Could you check a few things on this model? Use its own coordinates, in mm. A direction names the side the tool comes from. Give positions to 0.01 mm unless a question says otherwise; leave off trailing zeros. Order: outer loops, then holes, each group sorted by start corner. A loop starts at its lowest first (then second) coordinate and runs counter-clockwise, first axis right, second up. Notation, with made-up numbers: (46.25, -35) -> (92.25, -35) arc R16 ccw to (92.25, -28) -> close; hole circle Ø7 at (3.25, 25). An arc over 180 degrees is marked (long way). Answer as CSV lines item,"result". Start each with the question number.
(1) I want a section at A-A (y = 4.5). Please give me the cut outline in (x, z).
(2) Will these pins go through, and if not, where does the flat tip stop? pin 1 Ø1 at (x, y) = (-8.5, 5) entering from +Z; pin 2 Ø2 at (x, z) = (-15.25, -15.25) entering from -Y; pin 3 Ø0.7 at (x, y) = (10, -0.5) entering from -Z; pin 4 Ø6 at (x, z) = (-1.5, 5.5) entering from +Y.
(3) I want a section at C-C (y = 0). Give the number of separate pieces and of enclosed holes in the cut face, plus the area to 3 significant figures.
(4) I need wall thicknesses on L1, parallel to X at y = 2.5, z = -10; L2, parallel to X at y = -1.4, z = -10; L3, parallel to X at y = -0.2, z = -15.25. Which ranges of each line are inside material? Lowest first, please.
(5) I want a section at B-B (z = 5). Please give me the cut outline in (x, y).
(6) We'd pull the mould along Z, two halves only. Please class faces 1 (the face through (10.203, 0.024, -21.141)), 2 (the face through (9, 0, -24.5)), 3 (the face through (-12.46, 0.02, -11.44)): released by +Z, released by -Z, zero draft, split by the parting line, or undercut.
(7) On a 3-axis mill with a long thin cutter (end or side, diameter ignored), from which of +Z, -Z, +X, -X, +Y, -Y can I reach the whole of each face in a straight line? I mean faces 4 (the face through (-12, 6.7, 10)), 5 (the face through (-14, 0, -20)), 6 (the face through (10, 0, 12.85)), 7 (the face through (8.388, 4.235, 7.897)). Say none if no direction works.
```python
from build123d import *

# Parameters (mm, degrees)
BOSS_EXTRUDE1_DEPTH = 1.7
SKETCH2_R           = 1.65
CUT_EXTRUDE1_DEPTH  = 3.4
BOSS_EXTRUDE2_START = 5
SKETCH3_R           = 2.65
SKETCH3_R_2         = 1.65
BOSS_EXTRUDE2_DEPTH = 5
CUT_EXTRUDE2_START  = -0.5
CUT_EXTRUDE2_DEPTH  = 2.4


with BuildPart() as part:
    # Sketch1 → Boss-Extrude1 (new, symmetric)
    with BuildSketch(Plane(origin=(0, 0, 0), x_dir=(1, 0, 0), z_dir=(0, 1, 0))):
        with BuildLine():
            Line((-13, 20), (-15.757359313, 20))
            Line((-15.757359313, 20), (-20, 15.757359313))
            Line((-20, 15.757359313), (-20, -15.757359313))
            Line((-20, -15.757359313), (-15.757359313, -20))
            Line((-15.757359313, -20), (15.757359313, -20))
            Line((15.757359313, -20), (20, -15.757359313))
            Line((20, -15.757359313), (20, 15.757359313))
            Line((20, 15.757359313), (15.757359313, 20))
            Line((15.757359313, 20), (13, 20))
            ThreePointArc((13, 20), (10.171572875, 21.171572875), (9, 24))
            Line((9, 24), (9, 25))
            ThreePointArc((9, 25), (7.828427125, 27.828427125), (5, 29))
            Line((5, 29), (-5, 29))
            ThreePointArc((-5, 29), (-7.828427125, 27.828427125), (-9, 25))
            Line((-9, 25), (-9, 24))
            ThreePointArc((-9, 24), (-10.171572875, 21.171572875), (-13, 20))
        make_face()
    extrude(amount=BOSS_EXTRUDE1_DEPTH, both=True)

    # Sketch2 → Cut-Extrude1 (cut)
    with BuildSketch(Plane(origin=(0, 1.7, 0), x_dir=(1, 0, 0), z_dir=(0, 1, 0))):
        with Locations(Location((-10, 10, 0), (0, 0, 270))):
            Circle(SKETCH2_R)
        with Locations(Location((10, 10, 0), (0, 0, 270))):
            Circle(SKETCH2_R)
        with Locations(Location((-10, -10, 0), (0, 0, 270))):
            Circle(SKETCH2_R)
        with Locations(Location((10, -10, 0), (0, 0, 270))):
            Circle(SKETCH2_R)
        with Locations(Location((-15.25, -15.25, 0), (0, 0, 270))):
            Circle(SKETCH2_R)
        with Locations(Location((-15.25, 15.25, 0), (0, 0, 270))):
            Circle(SKETCH2_R)
        with Locations(Location((15.25, 15.25, 0), (0, 0, 270))):
            Circle(SKETCH2_R)
        with Locations(Location((15.25, -15.25, 0), (0, 0, 270))):
            Circle(SKETCH2_R)
    extrude(amount=-CUT_EXTRUDE1_DEPTH, mode=Mode.SUBTRACT)

    # Sketch3 → Boss-Extrude2 (add)
    # profile 1 of 4: a face of its own
    with BuildSketch(Plane(origin=(0, 1.7, 0), x_dir=(1, 0, 0), z_dir=(0, 1, 0)).offset(BOSS_EXTRUDE2_START)):
        with Locations(Location((-10, 10, 0), (0, 0, 270))):
            Circle(SKETCH3_R)
        with Locations(Location((-10, 10, 0), (0, 0, 270))):
            Circle(SKETCH3_R_2, mode=Mode.SUBTRACT)
    # profile 2 of 4: a face of its own
    with BuildSketch(Plane(origin=(0, 1.7, 0), x_dir=(1, 0, 0), z_dir=(0, 1, 0)).offset(BOSS_EXTRUDE2_START)):
        with Locations(Location((10, 10, 0), (0, 0, 270))):
            Circle(SKETCH3_R)
        with Locations(Location((10, 10, 0), (0, 0, 270))):
            Circle(SKETCH3_R_2, mode=Mode.SUBTRACT)
    # profile 3 of 4: a face of its own
    with BuildSketch(Plane(origin=(0, 1.7, 0), x_dir=(1, 0, 0), z_dir=(0, 1, 0)).offset(BOSS_EXTRUDE2_START)):
        with Locations(Location((10, -10, 0), (0, 0, 270))):
            Circle(SKETCH3_R)
        with Locations(Location((10, -10, 0), (0, 0, 270))):
            Circle(SKETCH3_R_2, mode=Mode.SUBTRACT)
    # profile 4 of 4: a face of its own
    with BuildSketch(Plane(origin=(0, 1.7, 0), x_dir=(1, 0, 0), z_dir=(0, 1, 0)).offset(BOSS_EXTRUDE2_START)):
        with Locations(Location((-10, -10, 0), (0, 0, 270))):
            Circle(SKETCH3_R)
        with Locations(Location((-10, -10, 0), (0, 0, 270))):
            Circle(SKETCH3_R_2, mode=Mode.SUBTRACT)
    extrude(amount=-BOSS_EXTRUDE2_DEPTH)

    # Sketch4 → Cut-Extrude2 (cut)
    with BuildSketch(Plane(origin=(0, 1.7, 0), x_dir=(1, 0, 0), z_dir=(0, 1, 0)).offset(CUT_EXTRUDE2_START)):
        Polygon((-6.709103466, 10), (-8.354551733, 12.85), (-11.645448267, 12.85), (-13.290896534, 10), (-11.645448267, 7.15), (-8.354551733, 7.15), align=None)
        Polygon((13.290896534, 10), (11.645448267, 12.85), (8.354551733, 12.85), (6.709103466, 10), (8.354551733, 7.15), (11.645448267, 7.15), align=None)
        Polygon((13.290896534, -10), (11.645448267, -7.15), (8.354551733, -7.15), (6.709103466, -10), (8.354551733, -12.85), (11.645448267, -12.85), align=None)
        Polygon((-6.709103466, -10), (-8.354551733, -7.15), (-11.645448267, -7.15), (-13.290896534, -10), (-11.645448267, -12.85), (-8.354551733, -12.85), align=None)
    extrude(amount=-CUT_EXTRUDE2_DEPTH, mode=Mode.SUBTRACT)


solid = part.part
```
Final values:
1,outline,"circle Ø5.3 at (-10, -10); circle Ø5.3 at (-10, 10); circle Ø5.3 at (10, -10); circle Ø5.3 at (10, 10); hole circle Ø3.3 at (-10, -10); hole circle Ø3.3 at (-10, 10); hole circle Ø3.3 at (10, -10); hole circle Ø3.3 at (10, 10)"
2,pin 1,"z = 12.45"
2,pin 2,"through"
2,pin 3,"z = -21.81"
2,pin 4,"y = 1.7"
3,separate pieces,"1"
3,enclosed holes,"8"
3,area,"1,580 mm²"
4,L1,"-12.65 to -11.65, -8.35 to -7.35, 7.35 to 8.35, 11.65 to 12.65"
4,L2,"-20 to -11.65, -8.35 to 8.35, 11.65 to 20"
4,L3,"-20 to -16.9, -13.6 to 13.6, 16.9 to 20"
5,outline,"(-20, -1.7) -> (20, -1.7) -> (20, 1.7) -> (-20, 1.7) -> close"
6,face 1,"released by -Z"
6,face 2,"zero draft"
6,face 3,"undercut"
7,face 4,"+Z, -Z, +X, -X, +Y"
7,face 5,"-Z, -X, +Y, -Y"
7,face 6,"none"
7,face 7,"+Y"
